Part model, mm, in its own coordinate system. Face numbers are marked on the shaded views. A direction names the side the tool comes from. Round coordinates to 2 decimals unless told otherwise and drop trailing zeros. Loops run counter-clockwise (first coordinate to the right, second up) from the corner with the lowest first, then second, coordinate; pieces in that order, holes last.
1) Drop flat-ended pins along their axis: P1, Ø1, axis at y = 7.5, z = -0.5, coming from the +X side; P2, Ø1, axis at x = 1.5, y = 5.5, coming from the +Z side; P3, Ø2, axis at x = 0, y = 10, coming from the -Z side (3 decimals); P4, Ø0.6, axis at x = 0, z = 3, coming from the -Y side. Give the stop position or say it passes through.
2) Band-saw the part on B-B, the plane x = 0. Write the cut outline in (y, z), then the cut area to 4 significant figures.
3) Band-saw the part on D-D, the plane y = 4. Write the cut outline in (x, z), then the cut area to 4 significant figures.
4) Probe line 1 (Y direction, x = 0.25, z = -0.5); line 2 (Y direction, x = -2, z = 1.75); line 3 (Z direction, x = 0.5, y = 6.5). List the from-to ranges inside material, lowest first.
5) Band-saw the part on A-A, the plane y = 10.4. Write the cut outline in (x, z), then the cut area to 3 significant figures.
6) Band-saw the part on C-C, the plane z = -2.5. State how many separate pieces and enclosed holes the cut face has, then the cut area to 3 significant figures.
7) 3-axis set-ups, long thin cutter, end or side, ignore diameter. For the marked faces 1, 2 and 3: which of +Z, -Z, +X, -X, +Y, -Y reach the whole face in a straight line?
8) Mould opens along Y. For the marked faces 4, 5 and 6 say: +Y half, -Y half, draft (parallel to the pull), parting line (faces both ways), or undercut.
Autodesk Inventor part; units mm, degrees
ref_plane "YZ Plane" through (0, 0, 0) normal (1, 0, 0) x (0, 1, 0)
ref_plane "XZ Plane" through (0, 0, 0) normal (0, 1, 0) x (-1, 0, 0)
ref_plane "XY Plane" through (0, 0, 0) normal (0, 0, 1) x (1, 0, 0)
sketch "スケッチ1" plane through (0, 0, 0) normal (0, 1, 0) x (-1, 0, 0)
  line L0 (3.5, 4.25) -> (-3.5, 4.25)
  line L1 (-3.5, 4.25) -> (-3.5, -4.25)
  line L2 (-3.5, -4.25) -> (3.5, -4.25)
  line L3 (3.5, -4.25) -> (3.5, 4.25)
  line L4 (3.5, 4.25) -> (-3.5, -4.25) construction
  line L5 (-3.5, 4.25) -> (3.5, -4.25) construction
  point P0 (0, 0)
  dimension "d0" = 7
  dimension "d1" = 8.5
extrude "押し出し1" add sketch "スケッチ1" along normal blind 15
sketch "スケッチ2" plane through (-3.5, 0, 4.25) normal (0, 0, 1) x (1, 0, 0)
  circle A0 centre (3.5, 4) radius 2.35
  line L0 (0, 0) -> (7, 0)
  line L1 (0, 0) -> (0, 15)
  circle A1 centre (3.5, 10.4) radius 2.6
  line L2 (0, 15) -> (7, 15)
  point P0 (3.5, 0)
  dimension "d4" = 4.7
  dimension "d5" = 4
  dimension "d6" = 3.5
  dimension "d7" = 5.2
  dimension "d8" = 4.6
  dimension "d9" = 3.5
extrude "押し出し2" cut sketch "スケッチ2" against normal blind 9
fillet "フィレット1" radius 2 1 edges at (3.5, 15, 0)
fillet "フィレット2" radius 2 1 edges at (-3.5, 15, 0)
sketch "スケッチ4" plane through (0, 0, 0) normal (0, -1, 0) x (1, 0, 0)
  line L0 (0, 6.3882) -> (0, -6.0661)
  line L1 (-5.5555, 5.25) -> (5.1337, 5.25)
  line L2 (-3.5, 4.25) -> (3.5, 4.25)
  point P0 (0, 0)
  dimension "d23" = 1
sketch "スケッチ6" plane through (-3.5, 0, 4.25) normal (0, 0, 1) x (1, 0, 0)
  line L0 (0, 0) -> (7, 0)
  line L1 (0, 0) -> (7, 0)
  line L2 (7, 0) -> (7, 7)
  line L3 (7, 7) -> (0, 7)
  line L4 (0, 7) -> (0, 0)
  point P0 (3.5, 0)
  dimension "d27" = 7
  dimension "d28" = 7
extrude "押し出し4" cut sketch "スケッチ6" against normal blind 2
sketch "スケッチ8" plane through (3.5, 0, -4.25) normal (0, 0, -1) x (-1, 0, 0)
  arc A0 (2, 7) -> (0, 5) centre (2, 5) ccw
  arc A1 (7, 5) -> (5, 7) centre (5, 5) ccw
  line L0 (0, 7) -> (7, 7) construction
  line L1 (0, 0) -> (7, 0) construction
  line L2 (0, 0) -> (0, 13) construction
  line L3 (7, 0) -> (7, 13) construction
  arc A2 (0, 9) -> (2, 7) centre (2, 9) ccw
  arc A3 (5, 7) -> (7, 9) centre (5, 9) ccw
  line L4 (0, 5) -> (0, 9)
  line L5 (7, 5) -> (7, 9)
  line L6 (7, 7) -> (7, 13)
  point P0 (3.5, 0)
  dimension "d33" = 2
  dimension "d34" = 7
extrude "押し出し5" cut sketch "スケッチ8" against normal blind 8.5
fillet "フィレット3" radius 2 2 edges at (1.5, 7, -1) (-1.5, 7, -1)
sketch "スケッチ9" plane through (-3.5, 0, 2.25) normal (0, 0, 1) x (1, 0, 0)
  arc A0 (7, 5) -> (6.7321, 6) centre (5, 5) ccw
  line L0 (7, 0) -> (7, 5)
  line L1 (7, 0) -> (0, 0)
  line L2 (0, 0) -> (0, 5)
  arc A1 (0.2679, 6) -> (0, 5) centre (2, 5) ccw
  arc A2 (0.2679, 6) -> (0.2679, 8) centre (-1.4641, 7) ccw
  arc A3 (0, 9) -> (0.2679, 8) centre (2, 9) ccw
  line L3 (0, 9) -> (0, 13)
  arc A4 (2, 15) -> (0, 13) centre (2, 13) ccw
  line L4 (5, 15) -> (2, 15)
  arc A5 (7, 13) -> (5, 15) centre (5, 13) ccw
  line L5 (7, 9) -> (7, 13)
  arc A6 (6.7321, 8) -> (7, 9) centre (5, 9) ccw
  arc A7 (6.7321, 8) -> (6.7321, 6) centre (8.4641, 7) ccw
  circle A8 centre (3.5, 10.4) radius 2.6
  circle A9 centre (3.5, 4) radius 2.35
  arc A10 (5, 7) -> (6.7321, 8) centre (5, 9) ccw
  line L6 (2, 7) -> (5, 7)
  arc A11 (0.2679, 8) -> (2, 7) centre (2, 9) ccw
  point P0 (3.5, 0)
properties part number "LED_mount"
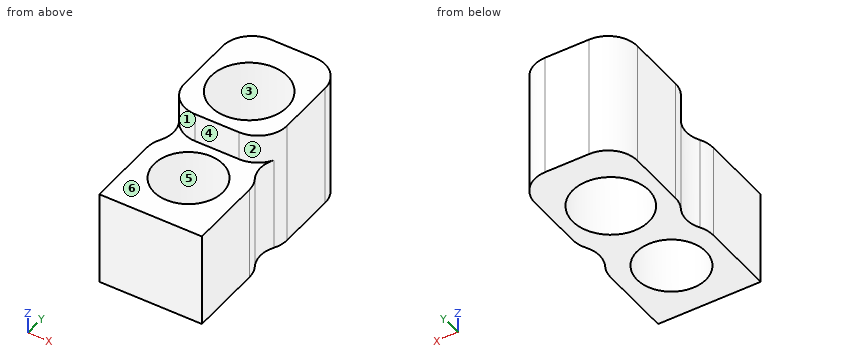
Reported:
1. P1: stops at x = 3.23
1. P2: stops at z = 2.25
1. P3: passes through
1. P4: stops at y = 7
2. outline: (0, -4.25) - (1.65, -4.25) - (1.65, 2.25) - (0, 2.25) - close; (6.35, -4.25) - (7.8, -4.25) - (7.8, 4.25) - (7, 4.25) - (7, 2.25) - (6.35, 2.25) - close; (13, -4.25) - (15, -4.25) - (15, 4.25) - (13, 4.25) - close
2. area: 38.75 mm2
3. outline: (-3.5, -4.25) - (-2.35, -4.25) - (-2.35, 2.25) - (-3.5, 2.25) - close; (2.35, -4.25) - (3.5, -4.25) - (3.5, 2.25) - (2.35, 2.25) - close
3. area: 14.95 mm2
4. line 1: y = 0 to 1.66, 6.34 to 7.81, 12.99 to 15
4. line 2: y = 0 to 2.77, 5.23 to 8.74, 12.06 to 14.94
4. line 3: z = -4.25 to 2.25
5. outline: (-3.5, -4.25) - (-2.6, -4.25) - (-2.6, 4.25) - (-3.5, 4.25) - close; (2.6, -4.25) - (3.5, -4.25) - (3.5, 4.25) - (2.6, 4.25) - close
5. area: 15.3 mm2
6. separate pieces: 1
6. enclosed holes: 2
6. area: 62.6 mm2
7. face 1: +Z, -X
7. face 2: +Z, +X
7. face 3: +Z, -Z
8. face 4: -Y half
8. face 5: undercut
8. face 6: draft
